Verification items for the finished model (mm, model axes). Face numbers are marked on the shaded views. A direction names the side the tool comes from. Round coordinates to 2 decimals unless told otherwise and drop trailing zeros. Loops run counter-clockwise (first coordinate to the right, second up) from the corner with the lowest first, then second, coordinate; pieces in that order, holes last. Notation, with made-up numbers: M -31.75,29 L 18.25,29 A23 cw 18.25,40 Z; hole C 55.5,-12.5 d8. An arc over 180 degrees is marked long. One line per item, written item: value.
from build123d import *

# Parameters (mm, degrees)
SKETCH1_W           = 30
SKETCH1_H           = 53
SKETCH1_R           = 8.5
BOSS_EXTRUDE1_DEPTH = 10


with BuildPart() as part:
    # Sketch1 → Boss-Extrude1 (new body)
    with BuildSketch(Plane(origin=(0, 0, 0), x_dir=(0, 0, -1), z_dir=(1, 0, 0))):
        with Locations((0, -13.5)):
            Rectangle(SKETCH1_W, SKETCH1_H)
        Circle(SKETCH1_R, mode=Mode.SUBTRACT)
        with BuildLine():
            Line((-5, -27.5), (-5, -32.5))
            ThreePointArc((-5, -32.5), (-7.5, -35), (-10, -32.5))
            Line((-10, -32.5), (-10, -27.5))
            ThreePointArc((-10, -27.5), (-7.5, -25), (-5, -27.5))
        make_face(mode=Mode.SUBTRACT)
        with BuildLine():
            Line((5, -27.5), (5, -32.5))
            ThreePointArc((5, -32.5), (7.5, -35), (10, -32.5))
            Line((10, -32.5), (10, -27.5))
            ThreePointArc((10, -27.5), (7.5, -25), (5, -27.5))
        make_face(mode=Mode.SUBTRACT)
    extrude(amount=BOSS_EXTRUDE1_DEPTH)


solid = part.part
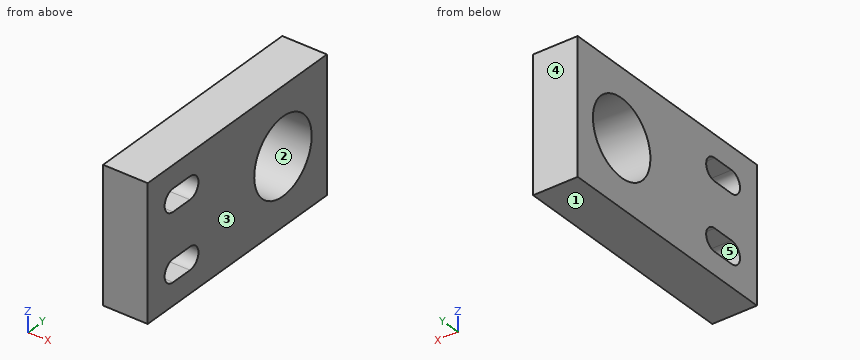
(1) Mould release check, pull along Z, two halves, no side actions. Record for the marked faces 1, 2 and 3: +Z half, -Z half, draft (parallel to the pull), parting line (faces both ways), or undercut.
Completed:
face 1: -Z half
face 2: undercut
face 3: draft
(2) Sectioned sample at A-A on z = -7.5. Enter the section's corners in (x, y).
Completed:
outline: M 0,-40 L 10,-40 L 10,-35 L 0,-35 Z; M 0,-25 L 10,-25 L 10,-4 L 0,-4 Z; M 0,4 L 10,4 L 10,13 L 0,13 Z
(3) Sectioned sample at D-D on z = 0. Enter the section's corners in (x, y), and give its area (3 significant figures).
Completed:
outline: M 0,-40 L 10,-40 L 10,-8.5 L 0,-8.5 Z; M 0,8.5 L 10,8.5 L 10,13 L 0,13 Z
area: 360 mm^2
(4) Tool access check on the marked faces 4 and 5. Record the directions out of +Z, -Z, +X, -X, +Y, -Y that give a thin tool (end or side, any length) a straight path to the whole face; none if there is none.
Completed:
face 4: +Z, -Z, +X, -X, +Y
face 5: +X, -X
(5) Thickness scan on L1, parallel to Y at x = 3.75, z = 0; L2, parallel to Y at x = 4.5, z = -7; L3, parallel to Y at x = 7.75, z = 5.25. Record the ranges inside material, lowest first. Write a range as from..to.
Completed:
L1: y = -40..-8.5, 8.5..13
L2: y = -40..-34.95, -25.05..-4.82, 4.82..13
L3: y = -40..-33.59, -26.41..-6.68, 6.68..13
(6) Sectioned sample at B-B on x = 3. Enter the section's corners in (y, z).
Completed:
outline: M -40,-15 L 13,-15 L 13,15 L -40,15 Z; hole M -32.5,-10 L -27.5,-10 A2.5 ccw -27.5,-5 L -32.5,-5 A2.5 ccw Z; hole M -32.5,5 L -27.5,5 A2.5 ccw -27.5,10 L -32.5,10 A2.5 ccw Z; hole C 0,0 d17
(7) Sectioned sample at C-C on y = 0. Enter the section's corners in (x, z).
Completed:
outline: M 0,-15 L 10,-15 L 10,-8.5 L 0,-8.5 Z; M 0,8.5 L 10,8.5 L 10,15 L 0,15 Z
